Autodesk Inventor part; units mm, degrees
ref_plane "YZ Plane" through (0, 0, 0) normal (1, 0, 0) x (0, 1, 0)
ref_plane "XZ Plane" through (0, 0, 0) normal (0, 1, 0) x (-1, 0, 0)
ref_plane "XY Plane" through (0, 0, 0) normal (0, 0, 1) x (1, 0, 0)
sketch "スケッチ1" plane through (0, 0, 0) normal (0, 0, 1) x (1, 0, 0)
  line L0 (-17, -52.5) -> (17, -52.5) construction
  line L1 (17, -52.5) -> (17, 52.5) construction
  line L2 (17, 52.5) -> (-17, 52.5) construction
  line L3 (-17, 52.5) -> (-17, -52.5) construction
  line L4 (-17, -52.5) -> (17, 52.5) construction
  line L5 (17, -52.5) -> (-17, 52.5) construction
  line L6 (-17, 34.6) -> (-17, 52.5)
  line L7 (-17, 52.5) -> (17, 52.5)
  line L8 (17, 52.5) -> (17, 34.6)
  line L9 (-17, -34.6) -> (-17, -52.5)
  line L10 (-17, -52.5) -> (17, -52.5)
  line L11 (17, -52.5) -> (17, -34.6)
  line L12 (-17, 32.5) -> (-22, 32.5)
  line L13 (-22, 32.5) -> (-22, -32.5)
  line L14 (-22, -32.5) -> (-17, -32.5)
  line L15 (17, 32.5) -> (22, 32.5)
  line L16 (22, 32.5) -> (22, -32.5)
  line L17 (22, -32.5) -> (17, -32.5)
  arc A0 (-17, 32.5) -> (-17, 34.6) centre (-17, 33.55) ccw
  arc A1 (-17, -34.6) -> (-17, -32.5) centre (-17, -33.55) ccw
  arc A2 (17, 34.6) -> (17, 32.5) centre (17, 33.55) ccw
  arc A3 (17, -32.5) -> (17, -34.6) centre (17, -33.55) ccw
  line L18 (0, 0) -> (17, 0) construction
  line L19 (0, 0) -> (0, 52.5) construction
  line L20 (-12, 42.5) -> (12, 42.5) construction
  line L21 (12, 42.5) -> (12, -42.5) construction
  line L22 (12, -42.5) -> (-12, -42.5) construction
  line L23 (-12, -42.5) -> (-12, 42.5) construction
  circle A4 centre (-12, 42.5) radius 1.2
  circle A5 centre (12, 42.5) radius 1.2
  circle A6 centre (12, -42.5) radius 1.2
  circle A7 centre (-12, -42.5) radius 1.2
  point P0 (0, 42.5)
  point P1 (0, 0)
  dimension "d87" = 1.05
  dimension "d88" = 105
  dimension "d89" = 5
  dimension "d90" = 20
  dimension "d91" = 34
  dimension "d92" = 2.4
  dimension "d93" = 5
  dimension "d94" = 10
  dimension "d95" = 10
extrude "押し出し1" add sketch "スケッチ1" along normal blind 5
sketch "スケッチ2" plane through (0, 0, 5) normal (0, 0, 1) x (1, 0, 0)
  line L0 (-17, 52.5) -> (-17, 34.6)
  line L1 (17, 34.6) -> (17, 52.5)
  line L2 (-40.5884, 60.19) -> (-17, 60.19)
  line L3 (-17, 60.19) -> (-17, -101.7483)
  line L4 (-17, -101.7483) -> (-40.5884, -101.7483)
  line L5 (-40.5884, -101.7483) -> (-40.5884, 60.19)
  line L6 (53.5752, 90.4043) -> (17, 90.4043)
  line L7 (17, 90.4043) -> (17, -93.5321)
  line L8 (17, -93.5321) -> (53.5752, -93.5321)
  line L9 (53.5752, -93.5321) -> (53.5752, 90.4043)
  point P0 (0, 0)
extrude "押し出し2" cut sketch "スケッチ2" against normal blind 2.5
sketch "スケッチ3" plane through (0, 0, 5) normal (0, 0, 1) x (1, 0, 0)
  line L0 (17, -32.5) -> (17, 32.5)
  line L1 (17, 52.5) -> (-17, 52.5)
  line L2 (-17, 32.5) -> (-17, -32.5)
  line L3 (-17, -52.5) -> (17, -52.5)
  circle A0 centre (-12, -42.5) radius 1.2
  circle A1 centre (-12, 42.5) radius 1.2
  line L4 (-8, -48.5) -> (8, -48.5)
  line L5 (8, -48.5) -> (8, -36.5)
  line L6 (8, -36.5) -> (-8, -36.5)
  line L7 (-8, -36.5) -> (-8, -48.5)
  line L8 (-12, -31.5) -> (12, -31.5)
  line L9 (12, -31.5) -> (12, 31.5)
  line L10 (12, 31.5) -> (-12, 31.5)
  line L11 (-12, 31.5) -> (-12, -31.5)
  line L12 (-8, 36.5) -> (8, 36.5)
  line L13 (8, 36.5) -> (8, 48.5)
  line L14 (8, 48.5) -> (-8, 48.5)
  line L15 (-8, 48.5) -> (-8, 36.5)
  line L16 (0, 52.5) -> (0, -52.5) construction
  line L17 (-17, 0) -> (17, 0) construction
  point P0 (0, 0)
  point P1 (0, -31.5)
  dimension "d100" = 4
  dimension "d101" = 4
  dimension "d102" = 4
  dimension "d103" = 4
  dimension "d104" = 6
  dimension "d105" = 5
  dimension "d106" = 6
  dimension "d107" = 5
  dimension "d108" = 5
extrude "押し出し3" cut sketch "スケッチ3" against normal blind 10 contours L7 L6 L5 L4 | L11 L10 L9 L8 | L15 L14 L13 L12
fillet "フィレット1" radius 5 12 edges at (-8, 48.5, 2.5) (8, 48.5, 2.5) (-8, 36.5, 2.5) (8, 36.5, 2.5) (-12, 31.5, 2.5) (12, 31.5, 2.5) (12, -31.5, 2.5) (-12, -31.5, 2.5) (-8, -36.5, 2.5) (-8, -48.5, 2.5) (8, -48.5, 2.5) (8, -36.5, 2.5)
equation "\"d88\" = d83"
equation "\"d90\" = d84"
equation "\"d102\" = d101"
equation "\"d103\" = d100"
equation "\"d106\" = d104"
equation "\"d107\" = d105"
properties part number "コックピット_2_サブフレーム_5" material "アセタール樹脂、黒"
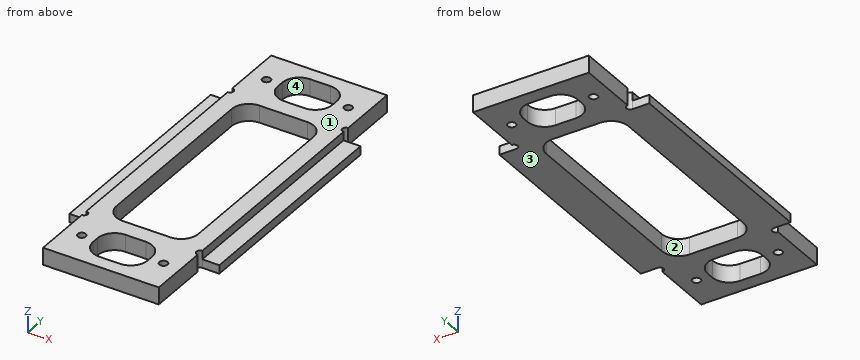
Could you check a few things on this model? Use its own coordinates, in mm. Face numbers are marked on the shaded views. A direction names the side the tool comes from. Round coordinates to 2 decimals unless told otherwise and drop trailing zeros. Write each loop counter-clockwise with the first axis right and the second up, starting at its lowest first coordinate (ties: lowest second). Pieces come first, ordered by that corner, then holes. Notation, with made-up numbers: (-2.5, 12) -> (54.5, 12) arc R20 ccw to (54.5, 34) -> close; hole circle Ø11 at (14, -32). An arc over 180 degrees is marked (long way). Use a Markdown table: item, result.
1. If we section it at C-C (z = 0.9): State how many separate pieces and enclosed holes the cut face has, then the cut area to 3 significant figures.
Answer key:
| item | result |
|---|---|
| separate pieces | 1 |
| enclosed holes | 7 |
| area | 2,360 mm^2 |
2. Which directions (+Z, -Z, +X, -X, +Y, -Y) give clear straight access to the entire face, cutting with the end or side of a thin tool? Please do the marked faces 1 and 2.
Answer key:
| item | result |
|---|---|
| face 1 | +Z, +X, -X, +Y, -Y |
| face 2 | +Z, -Z |
3. If we section it at B-B (y = -6): List the corners of the cut face in (x, z) for me, then the cut area to 3 significant figures.
Answer key:
| item | result |
|---|---|
| outline | (-22, 0) -> (-12, 0) -> (-12, 5) -> (-17, 5) -> (-17, 2.5) -> (-22, 2.5) -> close; (12, 0) -> (22, 0) -> (22, 2.5) -> (17, 2.5) -> (17, 5) -> (12, 5) -> close |
| area | 75.0 mm^2 |
4. Please list where these lines run through material, in increasing order: probe 1 along Y at (x, z) = (0, 2.6); probe 2 along X at (y, z) = (16.5, 1.1); probe 3 along Y at (x, z) = (-12.5, 1.3).
Answer key:
| item | result |
|---|---|
| probe 1 | y = -52.5 to -48.5, -36.5 to -31.5, 31.5 to 36.5, 48.5 to 52.5 |
| probe 2 | x = -22 to -12, 12 to 22 |
| probe 3 | y = -52.5 to -43.59, -41.41 to 41.41, 43.59 to 52.5 |
5. We'd pull the mould along X, two halves only. Please class the marked faces 3 and 4: +X half, -X half, draft (parallel to the pull), parting line (faces both ways), or undercut.
Answer key:
| item | result |
|---|---|
| face 3 | draft |
| face 4 | undercut |
6. If we section it at A-A (y = -42.5): List the corners of the cut face in (x, z) for me.
Answer key:
| item | result |
|---|---|
| outline | (-17, 0) -> (-13.2, 0) -> (-13.2, 5) -> (-17, 5) -> close; (-10.8, 0) -> (-8, 0) -> (-8, 5) -> (-10.8, 5) -> close; (8, 0) -> (10.8, 0) -> (10.8, 5) -> (8, 5) -> close; (13.2, 0) -> (17, 0) -> (17, 5) -> (13.2, 5) -> close |
7. For pin 1 Ø4 at (x, y) = (-12, 42.5) entering from +Z; pin 2 Ø2 at (x, z) = (20, 1.5) entering from +Y; pin 3 Ø1.6 at (y, z) = (-43, 2) entering from -X; pin 4 Ø2 at (y, z) = (-5.5, 4) entering from +X, each with a flat end and sliding along its axis, tell me the tip position at first contact or that it passes through.
Answer key:
| item | result |
|---|---|
| pin 1 | stops at z = 5 |
| pin 2 | stops at y = 32.5 |
| pin 3 | stops at x = -17 |
| pin 4 | stops at x = 17 |
